Geometry: see drawing. Coordinates: mm, zero at the bounding-box minimum. A direction names the side the tool comes from. Give positions to 0.01 mm unless a question says otherwise; leave off trailing zeros. Write each loop counter-clockwise with the first axis right and the second up, starting at its lowest first coordinate (ties: lowest second). Pieces come first, ordered by that corner, then holes. Notation, with made-up numbers: (-18, 7.25) -> (0, 7.25) arc R22 cw to (0, 26.25) -> close; hole circle Ø1 at (-34.5, -9). An arc over 180 degrees is marked (long way). Answer as a JSON object with one key per item and string values. Group by question number.
Item 1: Section query C-C on z = 1.25. Return the cut outline in (x, y) (1 decimal).
Item 2: Section query A-A on x = 4.8. Return the cut outline in (y, z) (1 decimal).
Item 3: Access query for the marked faces 4 and 5. Directions: +Z, -Z, +X, -X, +Y, -Y. A direction counts if a zero-diameter tool reaches every point of the face in a straight line with its end or side. Return the directions, or none.
Item 4: First-contact query: pin 1 Ø2 at (x, y) = (1, 2.5) entering from +Z; pin 2 Ø1 at (y, z) = (3.5, 2.5) entering from -X. Flat tips, straight axial feed; report the tip coordinate or a pass-through.
Item 5: Ray query, probe 1 along Z at (x, y) = (2.75, 3.4) (1 decimal); probe 2 along Y at (x, z) = (0.65, 1.25); probe 3 along X at (y, z) = (1.8, 3). Return the intervals inside material, ascending. Write a range as from..to.
Item 6: Pull-direction query (Z, two-part tool) for the marked faces 1, 2 and 3; classes: pulls with the +Z half, pulls with the -Z half, needs draft (parallel to the pull), parting line crosses it, or undercut.
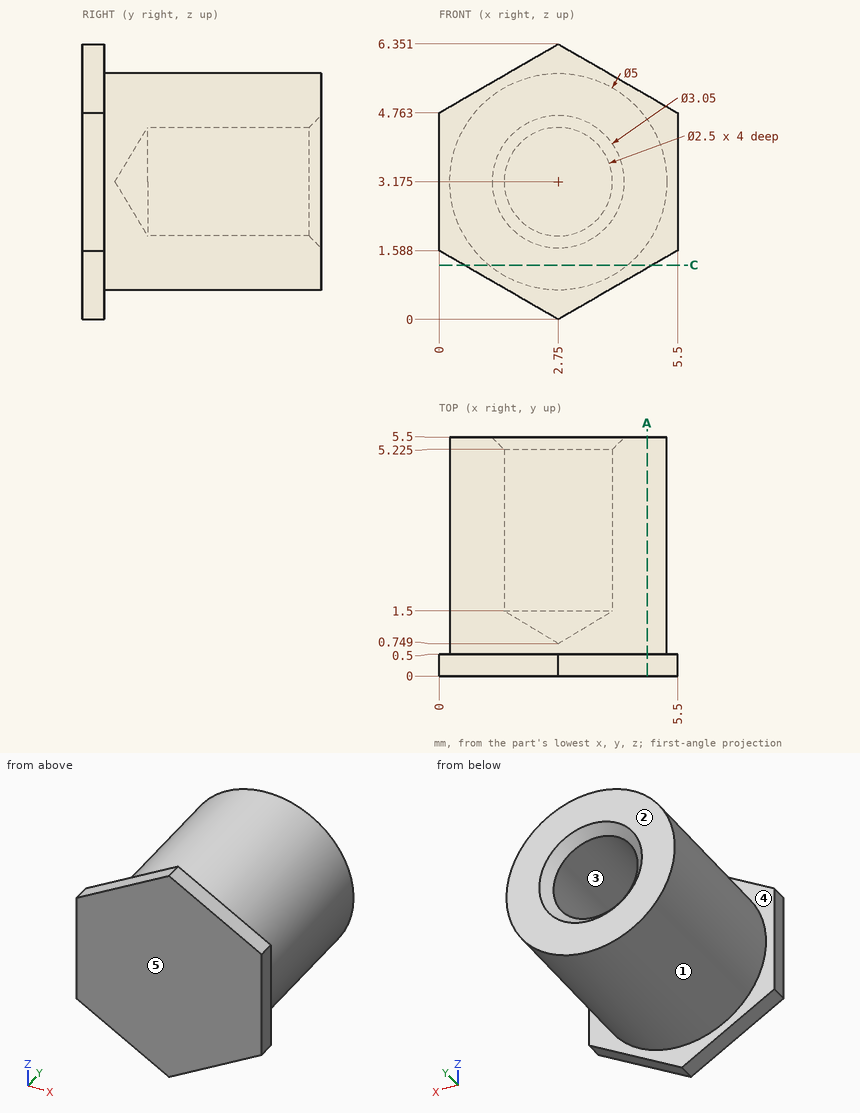
Worked answers:
{
 "1": {"outline": "(0.6, 0) -> (4.9, 0) -> (4.9, 0.5) -> (4.3, 0.5) -> (4.3, 5.5) -> (1.2, 5.5) -> (1.2, 0.5) -> (0.6, 0.5) -> close"},
 "2": {"outline": "(0, 1.2) -> (0.5, 1.2) -> (0.5, 1.7) -> (5.5, 1.7) -> (5.5, 4.6) -> (0.5, 4.6) -> (0.5, 5.2) -> (0, 5.2) -> close"},
 "3": {"face 4": "+Y", "face 5": "+Z, -Z, +X, -X, -Y"},
 "4": {"pin 1": "z = 5.56", "pin 2": "x = 0.26"},
 "5": {"probe 1": "0.7..1.9, 4.4..5.7", "probe 2": "0..0.5", "probe 3": "0.26..1.51, 3.99..5.24"},
 "6": {"face 1": "parting line crosses it", "face 2": "needs draft", "face 3": "undercut"}
}
